Model file for the job. Use its own axes, mm. Face numbers are marked on the shaded views. A direction names the side the tool comes from. Give positions to 0.01 mm unless a question says otherwise; leave off trailing zeros. Write each loop counter-clockwise with the first axis right and the second up, starting at its lowest first coordinate (ties: lowest second). Pieces come first, ordered by that corner, then holes. Notation, with made-up numbers: (54.25, -20.75) - (111.25, -20.75) arc R10 ccw to (111.25, -14.75) - close; hole circle Ø7 at (65.25, 28). An arc over 180 degrees is marked (long way). One line per item, written item: value. Start each with the question number.
(1) Probe L1, parallel to Y at x = 16, z = 17; L2, parallel to Y at x = -18, z = -26.5; L3, parallel to Z at x = 18.5, y = -10.5. List the from-to ranges inside material, lowest first.
(2) 3-axis set-ups, long thin cutter, end or side, ignore diameter. For the marked faces 5 and 6: which of +Z, -Z, +X, -X, +Y, -Y reach the whole face in a straight line?
(3) Cut at B-B, the plane z = -1.5. List the corners of the cut face in (x, y).
(4) Mould opens along X. For the marked faces 1, 2, 3 and 4 say: pulls with the +X half, pulls with the -X half, needs draft (parallel to the pull), parting line crosses it, or undercut.
(5) Cut at D-D, the plane y = -16. List the corners of the cut face in (x, z).
(6) Cut at C-C, the plane x = -18.5. List the corners of the cut face in (y, z), and give its area (3 significant figures).
(7) Cut at A-A, the plane y = -4. List the corners of the cut face in (x, z).
(8) Drop flat-ended pins along their axis: P1, Ø12, axis at x = -20, y = -7.5, coming from the +Z side; P2, Ø2, axis at x = 17, z = -18, coming from the -Y side; P3, Ø4, axis at x = -23.5, y = -13.5, coming from the -Z side. Give the stop position or say it passes through.
from build123d import *

# Parameters (mm, degrees)
F0_W          = 50
F0_H          = 65
F1_DEPTH      = 20
F3_DEPTH      = 25.4
F3_DEPTH_BACK = 25.4
F4_R          = 10
F6_DEPTH      = 10
F8_DEPTH      = 20
F10_DEPTH     = 65.0010001


with BuildPart() as f1:
    # F0 (on Front) → F1 (new body)
    with BuildSketch(Plane.XZ):
        Rectangle(F0_W, F0_H)
    extrude(amount=F1_DEPTH)

    # F2 (on face) → F3 (cut, two sides)
    with BuildSketch(Plane.XZ.offset(20)) as f3_sk:
        with BuildLine():
            Line((-7.9418579116, -14.0116587281), (9.2289298773, -14.0116587281))
            Line((9.2289298773, -14.0116587281), (9.2289298773, -6.7959995619))
            ThreePointArc((9.2289298773, -6.7959995619), (-0.2431108887, -13.3252146406), (-7.9418579116, -4.7765597701))
            Line((-7.9418579116, -4.7765597701), (-7.9418579116, -14.0116587281))
        make_face()
        with BuildLine():
            Line((9.2289298773, -4.5578256249), (9.2289298773, -6.7959995619))
            ThreePointArc((9.2289298773, -6.7959995619), (9.4266149422, -5.7397445697), (9.4928454099, -4.6671926975))
            ThreePointArc((9.4928454099, -4.6671926975), (0.8298353341, 4.0503304752), (-7.9418579116, -4.5578256249))
            Line((-7.9418579116, -4.5578256249), (9.2289298773, -4.5578256249))
        make_face()
        with BuildLine():
            ThreePointArc((-7.9418579116, -4.7765597701), (-0.2431108887, -13.3252146406), (9.2289298773, -6.7959995619))
            Line((9.2289298773, -6.7959995619), (9.2289298773, -4.5578256249))
            Line((9.2289298773, -4.5578256249), (-7.9418579116, -4.5578256249))
            Line((-7.9418579116, -4.5578256249), (-7.9418579116, -4.7765597701))
        make_face()
    extrude(amount=F3_DEPTH, mode=Mode.SUBTRACT)
    extrude(f3_sk.sketch, amount=-F3_DEPTH_BACK, mode=Mode.SUBTRACT)

    # F4
    f4_edges = [f1.edges().sort_by_distance(p)[0] for p in [
        (25, -10, 32.5),
        (-25, -10, 32.5),
    ]]
    fillet(f4_edges, radius=F4_R)

    # F5 (on face) → F6 (cut)
    with BuildSketch(Plane.XZ.offset(20)):
        Polygon((-20, -22.5), (-25, -22.5), (-25, -32.5), (-10, -32.5), align=None)
    extrude(amount=-F6_DEPTH, mode=Mode.SUBTRACT)

    # F7 (on face) → F8 (join)
    with BuildSketch(Plane.XZ.offset(20)):
        with BuildLine():
            add(Edge.make_bspline(
                [(-7.5, 22.5), (-7.5, 19.5948551827), (3.75, 21.0474275913), (15, 22.5), (3.75, 23.9525724087), (-7.5, 25.4051448173), (-7.5, 22.5)],
                knots=[0, 0, 0, 2.0943951024, 2.0943951024, 4.1887902048, 4.1887902048, 6.2831853072, 6.2831853072, 6.2831853072], degree=2, weights=[1, 0.5, 1, 0.5, 1, 0.5, 1]))
        make_face()
    extrude(amount=F8_DEPTH)

    # F9 (on face) → F10 (cut, through all)
    with BuildSketch(Plane(origin=(0, 0, -32.5), x_dir=(1, 0, 0), z_dir=(0, 0, -1))):
        with BuildLine():
            ThreePointArc((25, 15), (28.5355339059, 16.4644660941), (30, 20))
            ThreePointArc((30, 20), (25, 25), (20, 20))
            Line((20, 20), (25, 20))
            Line((25, 20), (25, 15))
        make_face()
    extrude(amount=-F10_DEPTH, mode=Mode.SUBTRACT)


solid = f1.part
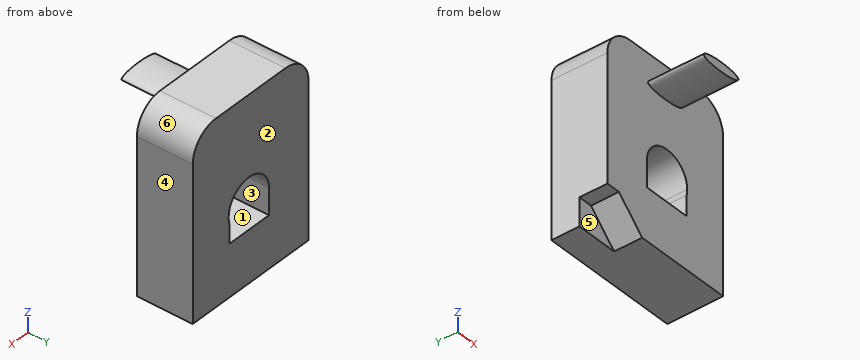
Answers follow:
1. L1: y = -20 to 0
1. L2: y = -10 to 0
1. L3: z = -32.5 to 31.87
2. face 5: -Z, -X, -Y
2. face 6: +Z, +X, +Y, -Y
3. outline: (-25, -20) - (-7.35, -20) - (-7.35, 0) - (-25, 0) - close; (8.9, -20) - (25, -20) - (25, 0) - (8.9, 0) - close
4. face 1: undercut
4. face 2: needs draft
4. face 3: undercut
4. face 4: pulls with the +X half
5. outline: (-25, -22.5) - (-20, -22.5) - (-10, -32.5) - (25, -32.5) - (25, 22.5) arc R10 ccw to (15, 32.5) - (-15, 32.5) arc R10 ccw to (-25, 22.5) - close; hole (-7.94, -14.01) - (9.23, -14.01) - (9.23, -6.8) arc R8.72 ccw (long way) to (-7.94, -4.56) - close
6. outline: (-20, -24) - (-10, -24) - (-10, -32.5) - (0, -32.5) - (0, 31.87) - (-20, 31.87) - close
6. area: 1,200 mm²
7. outline: (-25, -32.5) - (25, -32.5) - (25, 22.5) arc R10 ccw to (15, 32.5) - (-15, 32.5) arc R10 ccw to (-25, 22.5) - close; hole (-7.94, -14.01) - (9.23, -14.01) - (9.23, -6.8) arc R8.72 ccw (long way) to (-7.94, -4.56) - close
8. P1: stops at z = 32.5
8. P2: stops at y = -20
8. P3: stops at z = -22.5
